Build history of the part. All positions in model axes, mm. Face numbers are marked on the shaded views. A direction names the side the tool comes from. Round coordinates to 2 decimals unless told otherwise and drop trailing zeros. Order: outer loops, then holes, each group sorted by start corner. A loop starts at its lowest first (then second) coordinate and runs counter-clockwise, first axis right, second up. Notation, with made-up numbers: M -10.5,-37.75 L 45.5,-37.75 A20 ccw 45.5,-29.75 Z; hole C 50.5,-14.75 d7. An arc over 180 degrees is marked long. One line per item, written item: value. Start each with the question number.
Item 1: Band-saw the part on D-D, the plane x = -3.5. Write the cut outline in (y, z).
Item 2: Band-saw the part on A-A, the plane x = 0. Write the cut outline in (y, z) (3 decimals), then the cut area to 3 significant figures.
Item 3: Probe L1, parallel to X at y = 12.75, z = 0 (3 decimals); L2, parallel to Z at x = 0, y = 10.5 (3 decimals); L3, parallel to Y at x = 2.75, z = 4.25. List the from-to ranges inside material, lowest first.
Item 4: Band-saw the part on C-C, the plane z = -3.25. Write the cut outline in (x, y).
Item 5: Two-plate mould, pull along Z, no slides. Class the marked faces 1, 2 and 3: +Z half, -Z half, draft (parallel to the pull), parting line (faces both ways), or undercut.
Item 6: Pin check, flat tips, straight feed: pin 1 (5 mm diameter, centred on y = 3, z = 1.5, fed in from +X); pin 2 (3 mm diameter, centred on x = 0, z = 0, fed in from -Y); pin 3 (1 mm diameter, centred on y = 13.5, z = 4, fed in from -X); pin 4 (3 mm diameter, centred on x = 2.5, z = -1.5, fed in from -Y). Stop position of each tip, or through.
Item 7: Band-saw the part on B-B, the plane z = 0. Write the cut outline in (x, y) (3 decimals).
Item 8: Tool access for the marked faces 4, 5 and 6: list every direction of +Z, -Z, +X, -X, +Y, -Y with a clear straight run to the whole face (end or side of a thin tool).
```python
from build123d import *

# Parameters (mm, degrees)
SKETCH1_R               = 4.65
BOSS_EXTRUDE1_DEPTH     = 8
SKETCH2_W               = 10
SKETCH2_H               = 10
BOSS_EXTRUDE2_DEPTH     = 3
SKETCH3_R               = 4.655
BOSS_EXTRUDE3_DEPTH     = 8
CUT_EXTRUDE1_DEPTH      = 21.273134933
CUT_EXTRUDE1_DEPTH_BACK = 21.273134933
SKETCH4_R               = 2.655


with BuildPart() as part:
    # Sketch1 → Boss-Extrude1 (new body)
    with BuildSketch(Plane(origin=(0, 0, 0), x_dir=(1, 0, 0), z_dir=(0, 1, 0))):
        with Locations(Location((0, 0, 0), (0, 0, 270))):
            Circle(SKETCH1_R)
    extrude(amount=BOSS_EXTRUDE1_DEPTH)

    # Sketch2 → Boss-Extrude2 (add)
    with BuildSketch(Plane(origin=(0, 8, 0), x_dir=(1, 0, 0), z_dir=(0, 1, 0))):
        Rectangle(SKETCH2_W, SKETCH2_H)
    extrude(amount=BOSS_EXTRUDE2_DEPTH)

    # Sketch3 → Boss-Extrude3 (add)
    with BuildSketch(Plane(origin=(0, 11, 0), x_dir=(1, 0, 0), z_dir=(0, 1, 0))):
        with Locations(Location((0, 0, 0), (0, 0, 270))):
            Circle(SKETCH3_R)
    extrude(amount=BOSS_EXTRUDE3_DEPTH)

    # Sketch4 → Cut-Extrude1 (cut, two sides: drawn at the far end of the back side and taken through both)
    with BuildSketch(Plane(origin=(0, 19, 0), x_dir=(1, 0, 0), z_dir=(0, 1, 0)).offset(-CUT_EXTRUDE1_DEPTH_BACK)):
        with Locations(Location((0, 0, 0), (0, 0, 270))):
            Circle(SKETCH4_R)
    extrude(amount=CUT_EXTRUDE1_DEPTH + CUT_EXTRUDE1_DEPTH_BACK, mode=Mode.SUBTRACT)


solid = part.part
```
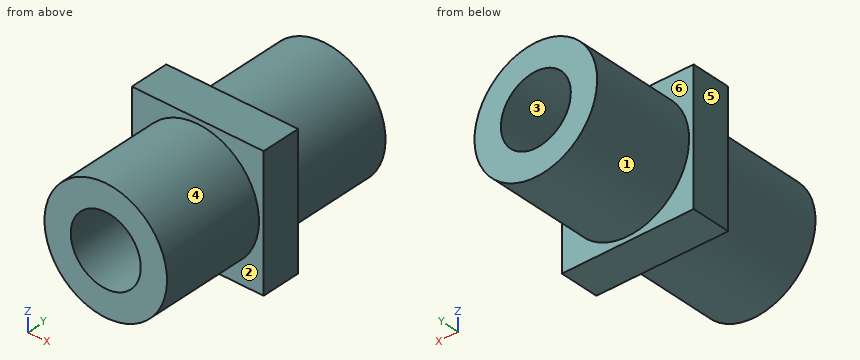
Output:
1. outline: M 0,-3.06 L 8,-3.06 L 8,-5 L 11,-5 L 11,-3.07 L 19,-3.07 L 19,3.07 L 11,3.07 L 11,5 L 8,5 L 8,3.06 L 0,3.06 Z
2. outline: M 0,-4.65 L 8,-4.65 L 8,-5 L 11,-5 L 11,-4.655 L 19,-4.655 L 19,-2.655 L 0,-2.655 Z; M 0,2.655 L 19,2.655 L 19,4.655 L 11,4.655 L 11,5 L 8,5 L 8,4.65 L 0,4.65 Z
2. area: 78.0 mm²
3. L1: x = -4.655 to -2.655, 2.655 to 4.655
3. L2: z = -5 to -2.655, 2.655 to 5
3. L3: y = 8 to 11
4. outline: M -5,8 L -3.33,8 L -3.33,0 L 3.33,0 L 3.33,8 L 5,8 L 5,11 L 3.33,11 L 3.33,19 L -3.33,19 L -3.33,11 L -5,11 Z
5. face 1: parting line
5. face 2: draft
5. face 3: undercut
6. pin 1: stops at x = 4.65
6. pin 2: passes through
6. pin 3: stops at x = -3.07
6. pin 4: stops at y = 0
7. outline: M -5,8 L -4.65,8 L -4.65,0 L -2.655,0 L -2.655,19 L -4.655,19 L -4.655,11 L -5,11 Z; M 2.655,0 L 4.65,0 L 4.65,8 L 5,8 L 5,11 L 4.655,11 L 4.655,19 L 2.655,19 Z
8. face 4: -Y
8. face 5: +Z, -Z, -X, +Y, -Y
8. face 6: +Y
